from build123d import *

# Parameters (mm, degrees)
F0_R     = 8.75
F1_DEPTH = 90
F3_DEPTH = 10
F5_R     = 4
F6_SIZE  = 5


# Not quite as in the source:
# - a fillet or chamfer that OpenCascade refuses, or shapes differently, is made with other operations: its cross-section is extruded or revolved along the edge and cut away or added


with BuildPart() as f1:
    # F0 (on Top) → F1 (new body)
    with BuildSketch(Plane.XY):
        Circle(F0_R)
        Polygon((3.75, 6.4951905284), (7.5, 0), (3.75, -6.4951905284), (-3.75, -6.4951905284), (-7.5, 0), (-3.75, 6.4951905284), align=None, mode=Mode.SUBTRACT)
    extrude(amount=F1_DEPTH)

    # F2 (on Top) → F3 (join)
    with BuildSketch(Plane.XY):
        with BuildLine():
            ThreePointArc((10, 40), (0, 50), (-10, 40))
            Line((-10, 40), (-10, 0))
            Line((-10, 0), (-10, -40))
            ThreePointArc((-10, -40), (0, -50), (10, -40))
            Line((10, -40), (10, 0))
            Line((10, 0), (10, 40))
        make_face()
    extrude(amount=-F3_DEPTH)

    # F4: chamfer of 5 on 1 edges, made by hand


with BuildPart() as f4_tool2:
    # F4_s3 → F4_t4 (revolve)
    with BuildSketch(Plane.XZ):
        Polygon((13.75, 0), (8.75, 5), (8.75, 0), align=None)
    revolve(axis=Axis((0, 0, 0), (0, 0, 1)))

    split(bisect_by=Plane.YZ.offset(10), keep=Keep.BOTTOM)

    split(bisect_by=Plane.YZ.offset(-10), keep=Keep.TOP)


with BuildPart() as f1_1:
    add(f1.part)

    # F4_t1: union F4_tool2
    add(f4_tool2.part)

    # F5
    f5_edges = [f1_1.edges().sort_by_distance(p)[0] for p in [
        (0, -13.75, 0),
        (0, 13.75, 0),
        (-8.75, 0, 5),
    ]]
    fillet(f5_edges, radius=F5_R)

    # F6
    f6_edges = [f1_1.edges().sort_by_distance(p)[0] for p in [
        (10, 0, -10),
    ]]
    chamfer(f6_edges, length=F6_SIZE)


solid = f1_1.part
Work out the finished part from the listing and answer in its coordinate system (mm). A direction names the side the tool comes from. Coordinates: 2 decimals unless noted, no trailing zeros. Loops run counter-clockwise (first coordinate to the right, second up) from the corner with the lowest first, then second, coordinate; pieces in that order, holes last. Notation, with made-up numbers: (-5.5, 57.5) -> (48.5, 57.5) arc R29 ccw to (48.5, 84.5) -> close; hole circle Ø6 at (17, -25.75). An arc over 180 degrees is marked (long way). Answer as CSV lines item,"result".
1) Straight lines are drawn through the part: probe 1 along Y at (x, z) = (0.5, 85.5); probe 2 along Z at (x, y) = (3.75, -21); probe 3 along Y at (x, z) = (7.25, 77). For each, find the intervals that lie inside material, in ascending order.
A:
probe 1,"y = -8.74 to -6.5, 6.5 to 8.74"
probe 2,"z = -10 to 0"
probe 3,"y = -4.9 to -0.43, 0.43 to 4.9"
2) For a pull along Y with two mould halves and no side action, classify faces 1 (the face through (7, -1, -8)), 2 (the face through (-5.6, -3.29, 44.37)), 3 (the face through (-6.944, -5.324, 47.745)) as released by +Y, released by -Y, zero draft, split by the parting line, or undercut.
A:
face 1,"zero draft"
face 2,"undercut"
face 3,"split by the parting line"
3) The part is cut by section A-A (z = 29). Give the vertices of the cut face in (x, y).
A:
outline,"circle Ø17.5 at (0, 0); hole (-7.5, 0) -> (-3.75, -6.5) -> (3.75, -6.5) -> (7.5, 0) -> (3.75, 6.5) -> (-3.75, 6.5) -> close"
4) The part is cut by section B-B (y = -36). Give the vertices of the cut face in (x, z), and give its area (3 significant figures).
A:
outline,"(-10, -5) -> (-5, -10) -> (5, -10) -> (10, -5) -> (10, 0) -> (-10, 0) -> close"
area,"175 mm²"
5) For faces 4 (the face through (0, 6.495, 44)), 5 (the face through (10, -1, -3)), determine the directions among +Z, -Z, +X, -X, +Y, -Y from which every point of the face is accessible in a straight line to the end or side of a thin tool.
A:
face 4,"+Z"
face 5,"+Z, -Z, +X, +Y, -Y"
6) Flat-ended cylindrical pins translate along their axes: pin 1 (10 mm diameter, centred on x = 4.5, y = -8.5, fed in from +Z); pin 2 (12 mm diameter, centred on x = 8, z = 69, fed in from +Y); pin 3 (10 mm diameter, centred on x = 6, z = 7.5, fed in from +Y); pin 4 (10 mm diameter, centred on x = 4.5, y = 34.5, fed in from +Z). Find the tip coordinate at first contact, or state that the pin passes through.
A:
pin 1,"stops at z = 90"
pin 2,"stops at y = 8.52"
pin 3,"stops at y = 10.07"
pin 4,"stops at z = 0"
